Source: CAD feature listing. Evaluate the final solid. Frame: model axes, mm. Face numbers are marked on the shaded views. A direction names the side the tool comes from. Coordinates: 2 decimals unless noted, no trailing zeros. Order: outer loops, then holes, each group sorted by start corner. A loop starts at its lowest first (then second) coordinate and runs counter-clockwise, first axis right, second up. Notation, with made-up numbers: (7, 64.25) -> (52, 64.25) arc R26 ccw to (52, 96.25) -> close; hole circle Ø6 at (37.5, -18). An arc over 180 degrees is marked (long way). Put each result on its own line as item: value.
from build123d import *

# Parameters (mm, degrees)
BOSS_EXTRU_1_DEPTH           = 25
ENL_V_MAT_EXTRU_1_DEPTH      = 50.203658401
ENL_V_MAT_EXTRU_1_DEPTH_BACK = 50.203658401
ESQUISSE2_R                  = 2


with BuildPart() as part:
    # Esquisse1 → Boss.-Extru.1 (new body)
    with BuildSketch(Plane.XY):
        Polygon((0, 0), (20, 0), (20, -14), (40, -14), (40, 8), (0, 8), align=None)
    extrude(amount=BOSS_EXTRU_1_DEPTH)

    # Esquisse2 → Enlèv. mat.-Extru.1 (cut, two sides: drawn at the far end of the back side and taken through both)
    with BuildSketch(Plane.XZ.offset(-ENL_V_MAT_EXTRU_1_DEPTH_BACK)):
        with Locations(Location((10, 12.5, 0), (0, 0, 270))):
            Circle(ESQUISSE2_R)
    extrude(amount=ENL_V_MAT_EXTRU_1_DEPTH + ENL_V_MAT_EXTRU_1_DEPTH_BACK, mode=Mode.SUBTRACT)


solid = part.part
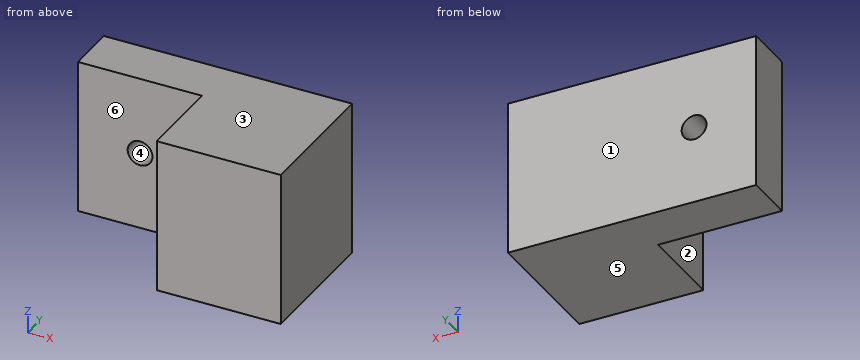
1. Cut plane B-B on z = 12.5. Output: boundary loops of the cut face in (x, y).
Numbers:
outline: (0, 0) -> (8, 0) -> (8, 8) -> (0, 8) -> close; (12, 0) -> (20, 0) -> (20, -14) -> (40, -14) -> (40, 8) -> (12, 8) -> close
2. Pull-direction query (Z, two-part tool) for the marked faces 3, 4, 5 and 6; classes: pulls with the +Z half, pulls with the -Z half, needs draft (parallel to the pull), parting line crosses it, or undercut.
Numbers:
face 3: pulls with the +Z half
face 4: undercut
face 5: pulls with the -Z half
face 6: needs draft
3. Set-up query: the marked faces 1 and 2. Return all of +Z, -Z, +X, -X, +Y, -Y with unobstructed straight access to the full face (end or side cutting, diameter ignored); none if empty.
Numbers:
face 1: +Z, -Z, +X, -X, +Y
face 2: +Z, -Z, -X, -Y
4. Ray query, line 1 along X through (y, z) = (2.5, 12.5); line 2 along Z through (x, y) = (10, 4); line 3 along X through (y, z) = (-11.25, 22.5). Return the intervals inside material, ascending.
Numbers:
line 1: x = 0 to 8, 12 to 40
line 2: z = 0 to 10.5, 14.5 to 25
line 3: x = 20 to 40
5. First-contact query: pin 1 (4 mm diameter, centred on y = -9, z = 12.5, fed in from -X); pin 2 (1.5 mm diameter, centred on x = 19, y = -9.5, fed in from +Z); pin 3 (10 mm diameter, centred on x = 6, z = 16, fed in from -Y). Flat tips, straight axial feed; report the tip coordinate or a pass-through.
Numbers:
pin 1: stops at x = 20
pin 2: passes through
pin 3: stops at y = 0
6. Cut plane A-A on x = 10. Output: boundary loops of the cut face in (y, z).
Numbers:
outline: (0, 0) -> (8, 0) -> (8, 10.5) -> (0, 10.5) -> close; (0, 14.5) -> (8, 14.5) -> (8, 25) -> (0, 25) -> close
7. Cut plane C-C on z = 19. Output: boundary loops of the cut face in (x, y).
Numbers:
outline: (0, 0) -> (20, 0) -> (20, -14) -> (40, -14) -> (40, 8) -> (0, 8) -> close
8. Cut plane D-D on y = -9. Output: boundary loops of the cut face in (x, z).
Numbers:
outline: (20, 0) -> (40, 0) -> (40, 25) -> (20, 25) -> close
